```python
from build123d import *

# Parameters (mm, degrees)
SKETCH1_W                       = 486.41
SKETCH1_H                       = 393.7
BOSS_EXTRUDE1_DEPTH             = 0.635
SKETCH2_R                       = 127
CUT_EXTRUDE1_DEPTH              = 313.89008841
BOSS_EXTRUDE2_REACH             = 314.888
SKETCH6_W                       = 1.27
SKETCH6_H                       = 9.525
BOSS_EXTRUDE2_DIRECTION_2_REACH = 314.888
FILLET1_R                       = 2.54


with BuildPart() as part:
    # Sketch1 → Boss-Extrude1 (new, symmetric)
    with BuildSketch(Plane(origin=(0, 0, 0), x_dir=(1, 0, 0), z_dir=(0, 1, 0))):
        Rectangle(SKETCH1_W, SKETCH1_H)
    extrude(amount=BOSS_EXTRUDE1_DEPTH, both=True)

    # Sketch2 → Cut-Extrude1 (cut, through all)
    with BuildSketch(Plane(origin=(0, 0.635, 0), x_dir=(1, 0, 0), z_dir=(0, 1, 0))):
        with Locations(Location((-25.4, 0, 0), (0, 0, 270))):
            Circle(SKETCH2_R)
    extrude(amount=-CUT_EXTRUDE1_DEPTH, mode=Mode.SUBTRACT)

    # Boss-Extrude2: up to this face of the body (flat: up to its plane)
    boss_extrude2_end = Plane(part.part.faces().sort_by_distance((0, 0, 196.85))[0])
    # Sketch6 → Boss-Extrude2 (add, up to the picked face)
    with BuildSketch(Plane.XY, mode=Mode.PRIVATE) as boss_extrude2_sk1:
        with Locations((-242.57, 4.1275)):
            Rectangle(SKETCH6_W, SKETCH6_H)
    boss_extrude2_tool1 = split(extrude(boss_extrude2_sk1.sketch, amount=BOSS_EXTRUDE2_REACH, mode=Mode.PRIVATE), bisect_by=boss_extrude2_end, keep=Keep.BOTH, mode=Mode.PRIVATE)
    add(boss_extrude2_tool1.solids().sort_by(Axis((-242.57, 4.1275, 0), (0, 0, 1)))[0])

    # Boss-Extrude2 direction 2: up to this face of the body (flat: up to its plane)
    boss_extrude2_direction_2_end = Plane(part.part.faces().sort_by_distance((0, 0, -196.85))[0])
    # Sketch6 → Boss-Extrude2 direction 2 (add, up to the picked face)
    with BuildSketch(Plane.XY, mode=Mode.PRIVATE) as boss_extrude2_direction_2_sk1:
        with Locations((-242.57, 4.1275)):
            Rectangle(SKETCH6_W, SKETCH6_H)
    boss_extrude2_direction_2_tool1 = split(extrude(boss_extrude2_direction_2_sk1.sketch, amount=-BOSS_EXTRUDE2_DIRECTION_2_REACH, mode=Mode.PRIVATE), bisect_by=boss_extrude2_direction_2_end, keep=Keep.BOTH, mode=Mode.PRIVATE)
    add(boss_extrude2_direction_2_tool1.solids().sort_by(Axis((-242.57, 4.1275, 0), (0, 0, -1)))[0])

    # Fillet1
    fillet1_edges = [part.edges().sort_by_distance(p)[0] for p in [
        (-241.935, 0.635, 0),
    ]]
    fillet(fillet1_edges, radius=FILLET1_R)


solid = part.part
```
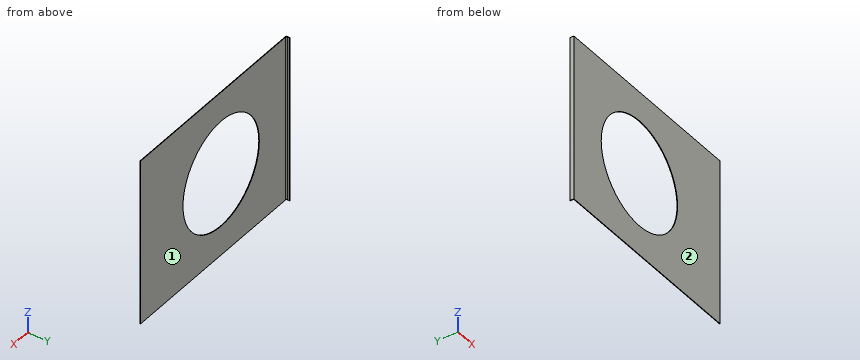
Can you work these out from the model? Positions are in its coordinate system, mm. Face numbers are marked on the shaded views. A direction names the side the tool comes from. Round coordinates to 2 decimals unless told otherwise and drop trailing zeros. Loops run counter-clockwise (first coordinate to the right, second up) from the corner with the lowest first, then second, coordinate; pieces in that order, holes last.
Item 1: Please list where these lines run through material, in increasing order: L1, parallel to X at y = 0.15, z = 0 (3 decimals); L2, parallel to Y at x = -73, z = 121 (3 decimals); L3, parallel to X at y = 5, z = -113.5 (3 decimals).
Item 2: Suppose I cut it at A-A, the plane z = 0. Write out the boundary of the cut face in (x, y) (3 decimals).
Item 3: Suppose I cut it at B-B, the plane x = -25.4. Write out the boundary of the cut face in (y, z) (3 decimals).
Item 4: Suppose I cut it at C-C, the plane z = 141. Write out the boundary of the cut face in (x, y) (3 decimals), then the cut area to 3 significant figures.
Item 5: Will these pins go through, and if not, where does the flat tip stop? pin 1 Ø10 at (x, z) = (107.5, 17) entering from +Y (3 decimals); pin 2 Ø4.5 at (y, z) = (5, 59.5) entering from +X.
Item 6: Suppose I cut it at D-D, the plane y = 5.5. Write out the boundary of the cut face in (x, z) (3 decimals), then the cut area to 3 significant figures.
Item 7: Which directions (+Z, -Z, +X, -X, +Y, -Y) give clear straight access to the entire face, cutting with the end or side of a thin tool? Please do the marked faces 1 and 2.
Reported:
1. L1: x = -243.205 to -152.4, 101.6 to 243.205
1. L2: y = -0.635 to 0.635
1. L3: x = -243.205 to -241.935
2. outline: (-243.205, -0.635) - (-152.4, -0.635) - (-152.4, 0.635) - (-239.395, 0.635) arc R2.54 cw to (-241.935, 3.175) - (-241.935, 8.89) - (-243.205, 8.89) - close; (101.6, -0.635) - (243.205, -0.635) - (243.205, 0.635) - (101.6, 0.635) - close
3. outline: (-0.635, -196.85) - (0.635, -196.85) - (0.635, -127) - (-0.635, -127) - close; (-0.635, 127) - (0.635, 127) - (0.635, 196.85) - (-0.635, 196.85) - close
4. outline: (-243.205, -0.635) - (243.205, -0.635) - (243.205, 0.635) - (-239.395, 0.635) arc R2.54 cw to (-241.935, 3.175) - (-241.935, 8.89) - (-243.205, 8.89) - close
4. area: 630 mm2
5. pin 1: stops at y = 0.635
5. pin 2: stops at x = -241.9
6. outline: (-243.205, -196.85) - (-241.935, -196.85) - (-241.935, 196.85) - (-243.205, 196.85) - close
6. area: 500 mm2
7. face 1: +Z, -Z, +X, +Y
7. face 2: +Z, -Z, +X, -X, -Y
